Input: dimensioned drawing with shaded views. Units: mm. Origin: part minimum x, y, z. A direction names the side the tool comes from. Round coordinates to 2 decimals unless told otherwise and drop trailing zeros. Write each loop counter-clockwise with the first axis right and the second up, starting at its lowest first coordinate (ties: lowest second). Pieces come first, ordered by that corner, then holes. Notation, with made-up numbers: (25.5, -30.75) -> (48.5, -30.75) arc R21 ccw to (48.5, -20.75) -> close; hole circle Ø1 at (-37, 10.25). An arc over 180 degrees is marked (long way). Return JSON: item names as keys, results as strings. Group by question number.
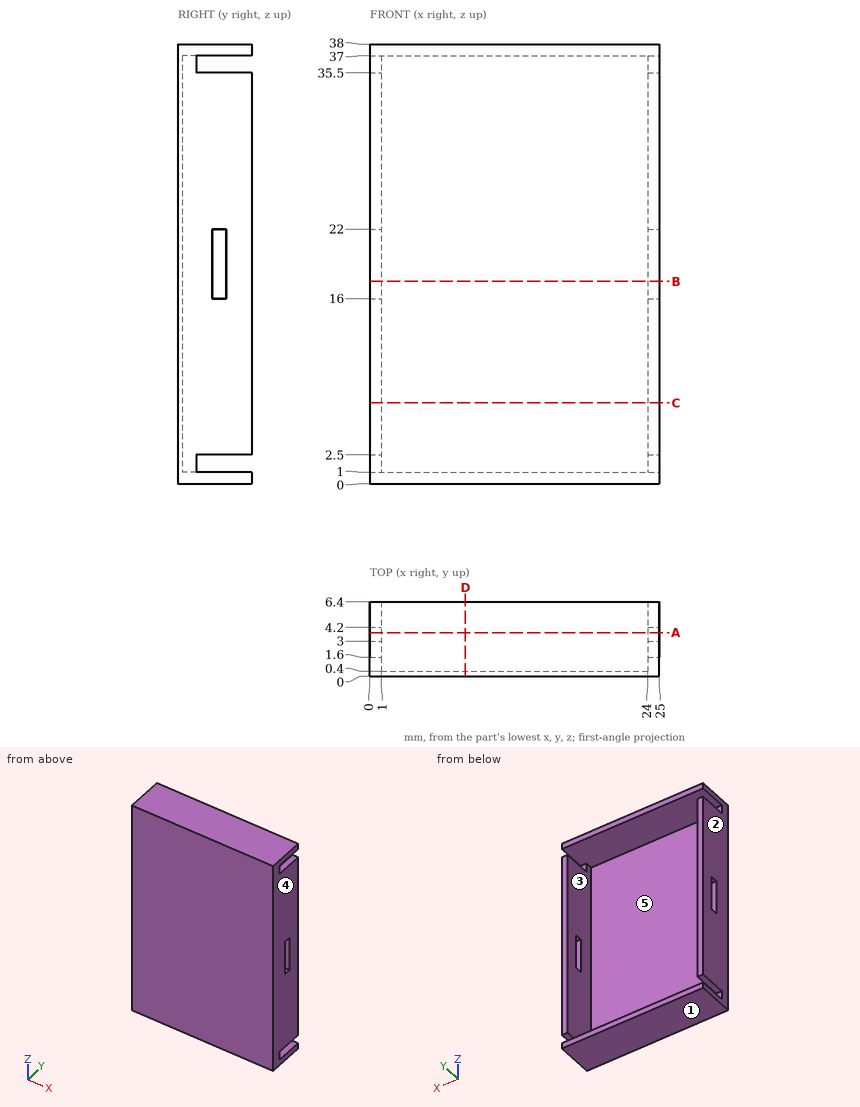
Item 1: Material intervals for probe 1 along Z at (x, y) = (22, 3); probe 2 along X at (y, z) = (1.5, 30); probe 3 along Y at (x, z) = (20.25, 28.5), sorted ascending.
Item 2: Cut plane C-C on z = 7. Output: boundary loops of the cut face in (x, y).
Item 3: Cut plane B-B on z = 17.5. Output: boundary loops of the cut face in (x, y), and give its area (3 significant figures).
Item 4: Cut plane D-D on x = 8.25. Output: boundary loops of the cut face in (y, z).
Item 5: Cut plane A-A on y = 3.75. Output: boundary loops of the cut face in (x, z).
Item 6: Set-up query: the marked faces 4 and 5. Return all of +Z, -Z, +X, -X, +Y, -Y with unobstructed straight access to the full face (end or side cutting, diameter ignored); none if empty.
Item 7: First-contact query: pin 1 Ø10 at (x, z) = (7.5, 16) entering from +Y; pin 2 Ø0.5 at (x, z) = (24.5, 2) entering from +Y. Flat tips, straight axial feed; report the tip coordinate or a pass-through.
Item 8: Pull-direction query (Z, two-part tool) for the marked faces 1, 2 and 3; classes: +Z half, -Z half, draft (parallel to the pull), parting line (faces both ways), or undercut.
Here are the results:
{
 "1": {"probe 1": "z = 0 to 1, 37 to 38", "probe 2": "x = 0 to 1, 24 to 25", "probe 3": "y = 0 to 0.4"},
 "2": {"outline": "(0, 0) -> (25, 0) -> (25, 6.4) -> (24, 6.4) -> (24, 0.4) -> (1, 0.4) -> (1, 6.4) -> (0, 6.4) -> close"},
 "3": {"outline": "(0, 0) -> (25, 0) -> (25, 3) -> (24, 3) -> (24, 0.4) -> (1, 0.4) -> (1, 3) -> (0, 3) -> close; (0, 4.2) -> (1, 4.2) -> (1, 6.4) -> (0, 6.4) -> close; (24, 4.2) -> (25, 4.2) -> (25, 6.4) -> (24, 6.4) -> close", "area": "19.6 mm^2"},
 "4": {"outline": "(0, 0) -> (6.4, 0) -> (6.4, 1) -> (0.4, 1) -> (0.4, 37) -> (6.4, 37) -> (6.4, 38) -> (0, 38) -> close"},
 "5": {"outline": "(0, 0) -> (25, 0) -> (25, 1) -> (0, 1) -> close; (0, 2.5) -> (1, 2.5) -> (1, 16) -> (0, 16) -> close; (0, 22) -> (1, 22) -> (1, 35.5) -> (0, 35.5) -> close; (0, 37) -> (25, 37) -> (25, 38) -> (0, 38) -> close; (24, 2.5) -> (25, 2.5) -> (25, 16) -> (24, 16) -> close; (24, 22) -> (25, 22) -> (25, 35.5) -> (24, 35.5) -> close"},
 "6": {"face 4": "+Z, -Z, +X, +Y, -Y", "face 5": "+Y"},
 "7": {"pin 1": "stops at y = 0.4", "pin 2": "stops at y = 1.6"},
 "8": {"face 1": "-Z half", "face 2": "draft", "face 3": "undercut"}
}
